from build123d import *

# Parameters (mm, degrees)
SKETCH037_W     = 96
SKETCH037_H     = 147
PAD011_DEPTH    = 10
SKETCH038_R     = 37.9
PAD012_DEPTH    = 2
SKETCH039_R     = 16
POCKET006_DEPTH = 8
SKETCH040_R     = 3
POCKET007_DEPTH = 4.001
SKETCH041_R     = 8.5
POCKET008_DEPTH = 8
SKETCH042_R     = 6
POCKET009_DEPTH = 4.001
SKETCH043_R     = 4.5
SKETCH043_R_2   = 6.5
POCKET010_DEPTH = 9
SKETCH044_R     = 4
SKETCH044_R_2   = 3
POCKET011_DEPTH = 3.001
SKETCH048_R     = 1.5
SKETCH048_R_2   = 1
POCKET012_DEPTH = 10.001
FILLET004_R     = 10


with BuildPart() as part:
    # Sketch037 → Pad011 (new body)
    with BuildSketch(Plane.XY):
        with Locations((-206.727857, -364.966475)):
            Rectangle(SKETCH037_W, SKETCH037_H)
    extrude(amount=PAD011_DEPTH)

    # Sketch038 (on Face6 of Pad011) → Pad012 (join)
    with BuildSketch(Plane.XY.offset(10)):
        with Locations((-206.727857, -339.466475)):
            Circle(SKETCH038_R)
    extrude(amount=PAD012_DEPTH)

    # Sketch039 (on Face8 of Pad012) → Pocket006 (cut)
    with BuildSketch(Plane.XY.offset(12)):
        with Locations((-206.727857, -358.416475)):
            Circle(SKETCH039_R)
    extrude(amount=-POCKET006_DEPTH, mode=Mode.SUBTRACT)

    # Sketch040 (on Face10 of Pocket006) → Pocket007 (cut, through all)
    with BuildSketch(Plane.XY.offset(4)):
        with Locations((-206.727857, -358.416475)):
            Circle(SKETCH040_R)
    extrude(amount=-POCKET007_DEPTH, mode=Mode.SUBTRACT)

    # Sketch041 (on Face8 of Pad012) → Pocket008 (cut)
    with BuildSketch(Plane.XY.offset(12)):
        with Locations((-231.877857, -339.466475)):
            Circle(SKETCH041_R)
    extrude(amount=-POCKET008_DEPTH, mode=Mode.SUBTRACT)

    # Sketch042 (on Face13 of Pocket008) → Pocket009 (cut, through all)
    with BuildSketch(Plane.XY.offset(4)):
        with Locations((-231.877857, -339.466475)):
            Circle(SKETCH042_R)
    extrude(amount=-POCKET009_DEPTH, mode=Mode.SUBTRACT)

    # Sketch043 (on Face8 of Pad012) → Pocket010 (cut)
    with BuildSketch(Plane.XY.offset(12)):
        with Locations((-192.827857, -339.466475)):
            Circle(SKETCH043_R)
        with Locations((-178.577857, -339.466475)):
            Circle(SKETCH043_R_2)
    extrude(amount=-POCKET010_DEPTH, mode=Mode.SUBTRACT)

    # Sketch044 (on Face18 of Pocket010) → Pocket011 (cut, through all)
    with BuildSketch(Plane.XY.offset(3)):
        with Locations((-178.577857, -339.466475)):
            Circle(SKETCH044_R)
        with Locations((-192.827857, -339.466475)):
            Circle(SKETCH044_R_2)
    extrude(amount=-POCKET011_DEPTH, mode=Mode.SUBTRACT)

    # Sketch048 (on Face5 of Pocket011) → Pocket012 (cut, through all)
    with BuildSketch(Plane.XY.offset(10)):
        with Locations((-244.727857, -301.466475)):
            Circle(SKETCH048_R)
        with Locations((-168.727857, -301.466475)):
            Circle(SKETCH048_R)
        with Locations((-168.727857, -428.466475)):
            Circle(SKETCH048_R)
        with Locations((-244.727857, -428.466475)):
            Circle(SKETCH048_R)
        with Locations((-214.611015, -276.454363)):
            Circle(SKETCH048_R_2)
        with Locations((-201.837814, -276.122591)):
            Circle(SKETCH048_R)
    extrude(amount=-POCKET012_DEPTH, mode=Mode.SUBTRACT)

    # Fillet004
    fillet004_edges = [part.edges().sort_by_distance(p)[0] for p in [
        (-254.727857, -438.466475, 5),
        (-158.727857, -438.466475, 5),
        (-254.727857, -291.466475, 5),
        (-158.727857, -291.466475, 5),
    ]]
    fillet(fillet004_edges, radius=FILLET004_R)


with BuildPart() as part_1:
    # Body010 placement: moved
    add(part.part.moved(Location((261.973389, 284.251869, 0))))


solid = part_1.part
Verification items for the finished model (mm, model axes). A direction names the side the tool comes from. Round coordinates to 2 decimals unless told otherwise and drop trailing zeros. Order: outer loops, then holes, each group sorted by start corner. A loop starts at its lowest first (then second) coordinate and runs counter-clockwise, first axis right, second up. Notation, with made-up numbers: (45.25, 11.25) -> (93.25, 11.25) arc R36 cw to (93.25, 47.25) -> close; hole circle Ø3 at (-2, 46.25). An arc over 180 degrees is marked (long way). Put each result on its own line as item: value.
1) Depth check by flat-ended pin: pin 1 (10.5 mm diameter, centred on x = 83.4, y = -55.21, fed in from +Z); pin 2 (4 mm diameter, centred on x = 93.25, y = -144.21, fed in from +Z). Enter the tip coordinate at first touch or a pass-through.
Final values:
pin 1: stops at z = 3
pin 2: stops at z = 10
2) Material ranges on line 1 (X direction, y = -144, z = 7.5); line 2 (Y direction, x = 55, z = 10.75); line 3 (Z direction, x = 13, y = -143.5), recorded low to high.
Final values:
line 1: x = 7.25 to 15.76, 18.73 to 91.76, 94.73 to 103.25
line 2: y = -93.11 to -90.16, -58.17 to -17.32
line 3: z = 0 to 10
3) Section check D-D (x = 63). Record the cut outline in (y, z).
Final values:
outline: (-154.21, 0) -> (-7.21, 0) -> (-7.21, 10) -> (-18.12, 10) -> (-18.12, 12) -> (-60.17, 12) -> (-60.17, 4) -> (-88.16, 4) -> (-88.16, 12) -> (-92.31, 12) -> (-92.31, 10) -> (-154.21, 10) -> close
4) Section check C-C (y = -82). Record the cut outline in (x, z).
Final values:
outline: (7.25, 0) -> (103.25, 0) -> (103.25, 10) -> (82.06, 10) -> (82.06, 12) -> (69.2, 12) -> (69.2, 4) -> (41.3, 4) -> (41.3, 12) -> (28.43, 12) -> (28.43, 10) -> (7.25, 10) -> close
5) Section check A-A (z = 7.75). Give the number of separate pieces and of enclosed holes in the cut face, then the cut area to 3 significant figures.
Final values:
separate pieces: 1
enclosed holes: 8
area: 12,800 mm^2
6) Section check B-B (x = 29). Record the cut outline in (y, z), then the cut area to 3 significant figures.
Final values:
outline: (-154.21, 0) -> (-61.11, 0) -> (-61.11, 4) -> (-63.64, 4) -> (-63.64, 12) -> (-82.56, 12) -> (-82.56, 10) -> (-154.21, 10) -> close; (-49.32, 0) -> (-7.21, 0) -> (-7.21, 10) -> (-27.87, 10) -> (-27.87, 12) -> (-46.79, 12) -> (-46.79, 4) -> (-49.32, 4) -> close
area: 1,400 mm^2
7) Set-up check for faces 1 (the flat face through (55, -154.215, 5)), 2 (the cylindrical face through (71.22, -59.21, 7.56)): record each of +Z, -Z, +X, -X, +Y, -Y from which the full face is reachable in a straight line by a thin tool's end or side.
Final values:
face 1: +Z, -Z, +X, -X, -Y
face 2: +Z
8) Mould release check, pull along X, two halves, no side actions. Record for faces 3 (the cylindrical face through (100.2, -151.4, 5.1)), 4 (the cylindrical face through (10.1, -10.22, 5.07)), 5 (the cylindrical face through (28.989, -46.787, 8.056)): +X half, -X half, draft (parallel to the pull), parting line (faces both ways), or undercut.
Final values:
face 3: +X half
face 4: -X half
face 5: undercut
